from build123d import *

# Parameters (mm, degrees)
F1_DEPTH = 63.5
F2_DEPTH = 25.4


with BuildPart() as f1:
    # F0 (on Front) → F1 (new body, symmetric)
    with BuildSketch(Plane.XZ):
        Polygon((41.275, -9.525), (41.275, 9.525), (22.225, 9.525), (-41.275, 9.525), (-41.275, -9.525), align=None)
    extrude(amount=F1_DEPTH, both=True)

    # F0 (on Front) → F2 (join)
    with BuildSketch(Plane.XZ):
        with BuildLine():
            Line((22.225, 9.525), (41.275, 9.525))
            Line((41.275, 9.525), (41.275, 27.0002))
            ThreePointArc((41.275, 27.0002), (45.92468, 38.22552), (57.15, 42.8752))
            Line((57.15, 42.8752), (60.325, 42.8752))
            Line((60.325, 42.8752), (60.325, 61.9252))
            Line((60.325, 61.9252), (57.15, 61.9252))
            add(Edge.make_bspline(
                [(53.938805, 61.777259), (55.022101, 61.84726), (56.092999, 61.896827), (57.15, 61.9252)],
                knots=[108.524772, 108.524772, 108.524772, 108.524772, 111.504536, 111.504536, 111.504536, 111.504536], degree=3))
            ThreePointArc((53.938805, 61.777259), (31.343929, 50.533205), (22.225, 27.0002))
            Line((22.225, 27.0002), (22.225, 9.525))
        make_face()
    extrude(amount=F2_DEPTH)


solid = f1.part
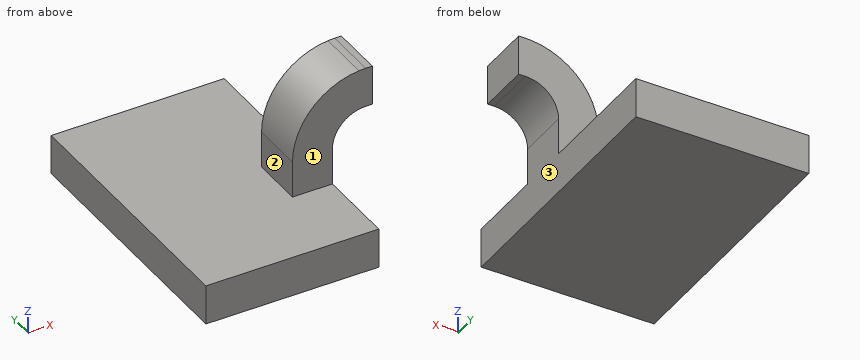
Here's how the part is built. I have some questions about the finished solid (model axes, mm). Face numbers are marked on the shaded views. A direction names the side the tool comes from. Round coordinates to 2 decimals unless told otherwise and drop trailing zeros. Write each loop counter-clockwise with the first axis right and the second up, starting at its lowest first coordinate (ties: lowest second). Pieces come first, ordered by that corner, then holes.
1. Suppose I cut it at C-C (z = 56). List the corners of the cut face in (x, y) for me (3 decimals).
2. Suppose I cut it at A-A (x = 34). List the corners of the cut face in (y, z) for me (3 decimals), and give its area (3 significant figures).
3. For the marked faces 1, 2 and 3, which set-ups out of +Z, -Z, +X, -X, +Y, -Y let a thin tool reach every point of the face, with its end or its side?
4. Will these pins go through, and if not, where does the flat tip stop? pin 1 Ø11.5 at (x, z) = (33.5, 28.5) entering from -Y; pin 2 Ø5 at (y, z) = (-7, 19) entering from +X (3 decimals); pin 3 Ø5 at (x, y) = (45, -21) entering from +Z.
5. I need wall thicknesses on L1, parallel to X at y = 0, z = -5.5 (3 decimals); L2, parallel to Z at x = 13, y = -7 (3 decimals); L3, parallel to Y at x = 39, z = 39. Which ranges of each line are inside material? Lowest first, please.
6. Suppose I cut it at B-B (y = 49). List the corners of the cut face in (x, z) for me (3 decimals), and give its area (3 significant figures).
Answer sheet:
1. outline: (37.688, -25.4) - (60.325, -25.4) - (60.325, 0) - (37.688, 0) - close
2. outline: (-63.5, -9.525) - (63.5, -9.525) - (63.5, 9.525) - (0, 9.525) - (0, 53.15) - (-25.4, 53.15) - (-25.4, 9.525) - (-63.5, 9.525) - close
2. area: 3,530 mm2
3. face 1: +Z, +X, -X, -Y
3. face 2: +Z, -X, +Y, -Y
3. face 3: -Z, +X, +Y, -Y
4. pin 1: stops at y = -25.4
4. pin 2: stops at x = 41.275
4. pin 3: stops at z = 60.57
5. L1: x = -41.275 to 41.275
5. L2: z = -9.525 to 9.525
5. L3: y = -25.4 to 0
6. outline: (-41.275, -9.525) - (41.275, -9.525) - (41.275, 9.525) - (-41.275, 9.525) - close
6. area: 1,570 mm2
